```python
from build123d import *

# Parameters (mm, degrees)
SKETCH1_W           = 32.735153169
SKETCH1_H           = 3.175
BOSS_EXTRUDE1_DEPTH = 3.175


with BuildPart() as part:
    # Sketch1 → Boss-Extrude1 (new body)
    with BuildSketch(Plane(origin=(0, 0, 0), x_dir=(0, 0, -1), z_dir=(1, 0, 0))):
        Polygon((-40.672653169, 9.525), (10.127346831, 9.525), (10.127346831, -13.316680621), (-40.672653169, -16.296041968), align=None)
        with Locations((-16.367576585, 1.5875)):
            Rectangle(SKETCH1_W, SKETCH1_H, mode=Mode.SUBTRACT)
    extrude(amount=-BOSS_EXTRUDE1_DEPTH)


solid = part.part
```
The model under review builds one solid part; all positions refer to its coordinate system, in mm. A direction names the side the tool comes from. Coordinates: 2 decimals unless noted, no trailing zeros. Order: outer loops, then holes, each group sorted by start corner. A loop starts at its lowest first (then second) coordinate and runs counter-clockwise, first axis right, second up. Notation, with made-up numbers: M 69.25,51.5 L 127.25,51.5 A28 ccw 127.25,72.5 Z; hole C 10,-34 d1. An arc over 180 degrees is marked long. One line per question, with ' | ' between items.
(1) Add section C-C, the plane z = 12. Write out the cut boundary in (x, y) (3 decimals).
Geometry results:
outline: M -3.175,-14.614 L 0,-14.614 L 0,0 L -3.175,0 Z; M -3.175,3.175 L 0,3.175 L 0,9.525 L -3.175,9.525 Z
(2) Insertion check: pin 1 (1.5 mm diameter, centred on y = -5.5, z = 29.5, fed in from +X). The pin has a flat end and moves straight along its axis. Give the tip position at first contact, or say it passes through.
Geometry results:
pin 1: stops at x = 0
(3) Add section D-D, the plane z = -3. Write out the cut boundary in (x, y) (3 decimals), then the cut area to 3 significant figures.
Geometry results:
outline: M -3.175,-13.735 L 0,-13.735 L 0,9.525 L -3.175,9.525 Z | area: 73.8 mm²
(4) Machinability: for faces 1 (the face through (-2, -2, -10.127)), 2 (the face through (-2, 3.175, 17)), which of the approach directions +Z, -Z, +X, -X, +Y, -Y give a long, thin tool a straight path to every point of the face, cutting with its end or side? Answer none if there is none.
Geometry results:
face 1: -Z, +X, -X, +Y, -Y | face 2: +X, -X
(5) The part is to be moulded in two halves that separate along Y. For faces 3 (the face through (-2, 9.525, 16)), 4 (the face through (-1.565, -14.786, 14.917)), 5 (the face through (-2, 0, 17)), 6 (the face through (-2, -4, 40.673)), say which applies: +Y half, -Y half, draft (parallel to the pull), parting line (faces both ways), or undercut.
Geometry results:
face 3: +Y half | face 4: -Y half | face 5: undercut | face 6: draft
(6) Add section A-A, the plane x = -1.8. Write out the cut boundary in (y, z) (3 decimals).
Geometry results:
outline: M -16.296,40.673 L -13.317,-10.127 L 9.525,-10.127 L 9.525,40.673 Z; hole M 0,0 L 3.175,0 L 3.175,32.735 L 0,32.735 Z
(7) Add section B-B, the plane z = 25. Write out the cut boundary in (x, y) (3 decimals).
Geometry results:
outline: M -3.175,-15.377 L 0,-15.377 L 0,0 L -3.175,0 Z; M -3.175,3.175 L 0,3.175 L 0,9.525 L -3.175,9.525 Z
(8) For probe 1 along Z at (x, y) = (-1.55, 1.25); probe 2 along Y at (x, z) = (-0.45, 21) (3 decimals); probe 3 along Y at (x, z) = (-2.5, 25) (3 decimals), list the stretches that pass through material, from the lowest coordinate up. Write a range as from..to.
Geometry results:
probe 1: z = -10.13..0, 32.74..40.67 | probe 2: y = -15.142..0, 3.175..9.525 | probe 3: y = -15.377..0, 3.175..9.525
